```python
from build123d import *

# Parameters (mm, degrees)
SKETCH1_W           = 60
SKETCH1_H           = 60
SKETCH1_R           = 28
SKETCH1_R_2         = 2.5
BOSS_EXTRUDE1_DEPTH = 7.5
SKETCH2_W           = 83.422483418
SKETCH2_H           = 79.797227822
SKETCH2_R           = 30
CUT_EXTRUDE1_DEPTH  = 2.5
BOSS_EXTRUDE2_START = -2
BOSS_EXTRUDE2_DEPTH = 2
FILLET1_R           = 3
FILLET2_R           = 5


with BuildPart() as part:
    # Sketch1 → Boss-Extrude1 (new, symmetric)
    with BuildSketch(Plane.XY):
        Rectangle(SKETCH1_W, SKETCH1_H)
        Circle(SKETCH1_R, mode=Mode.SUBTRACT)
        with Locations((25, 25)):
            Circle(SKETCH1_R_2, mode=Mode.SUBTRACT)
        with Locations((-25, 25)):
            Circle(SKETCH1_R_2, mode=Mode.SUBTRACT)
        with Locations((-25, -25)):
            Circle(SKETCH1_R_2, mode=Mode.SUBTRACT)
        with Locations((25, -25)):
            Circle(SKETCH1_R_2, mode=Mode.SUBTRACT)
    extrude(amount=BOSS_EXTRUDE1_DEPTH, both=True)

    # Sketch2 → Cut-Extrude1 (cut, symmetric)
    with BuildSketch(Plane.XY):
        Rectangle(SKETCH2_W, SKETCH2_H)
        Circle(SKETCH2_R, mode=Mode.SUBTRACT)
    extrude(amount=CUT_EXTRUDE1_DEPTH, both=True, mode=Mode.SUBTRACT)

    # Sketch3 → Boss-Extrude2 (add)
    with BuildSketch(Plane.XY.offset(7.5).offset(BOSS_EXTRUDE2_START)):
        with BuildLine():
            Line((14.986146269, -0.644530834), (22.978250586, -16))
            ThreePointArc((22.978250586, -16), (23.61864626, -15.038601957), (24.218842251, -14.051607738))
            Line((24.218842251, -14.051607738), (13.465479299, 6.609150267))
            Line((13.465479299, 6.609150267), (13.13845395, 7.237473855))
            ThreePointArc((13.13845395, 7.237473855), (7.905893272, 12.747425292), (0.644530834, 14.986146269))
            Line((0.644530834, 14.986146269), (16, 22.978250586))
            ThreePointArc((16, 22.978250586), (15.038601957, 23.61864626), (14.051607738, 24.218842251))
            Line((14.051607738, 24.218842251), (-7.237473855, 13.13845395))
            ThreePointArc((-7.237473855, 13.13845395), (-12.747425292, 7.905893272), (-14.986146269, 0.644530834))
            Line((-14.986146269, 0.644530834), (-22.978250586, 16))
            ThreePointArc((-22.978250586, 16), (-23.61864626, 15.038601957), (-24.218842251, 14.051607738))
            Line((-24.218842251, 14.051607738), (-13.465479299, -6.609150267))
            Line((-13.465479299, -6.609150267), (-13.13845395, -7.237473855))
            ThreePointArc((-13.13845395, -7.237473855), (-7.905893272, -12.747425292), (-0.644530834, -14.986146269))
            Line((-0.644530834, -14.986146269), (-16, -22.978250586))
            ThreePointArc((-16, -22.978250586), (-15.038601957, -23.61864626), (-14.051607738, -24.218842251))
            Line((-14.051607738, -24.218842251), (6.609150267, -13.465479299))
            Line((6.609150267, -13.465479299), (7.237473855, -13.13845395))
            ThreePointArc((7.237473855, -13.13845395), (12.747425292, -7.905893272), (14.986146269, -0.644530834))
        make_face()
    extrude(amount=BOSS_EXTRUDE2_DEPTH)

    # Fillet1
    fillet1_edges = [part.edges().sort_by_distance(p)[0] for p in [
        (24.218842251, -14.051607738, 6.5),
        (22.978250586, -16, 6.5),
        (14.986146269, -0.644530834, 6.5),
        (-14.051607738, -24.218842251, 6.5),
        (-16, -22.978250586, 6.5),
        (-0.644530834, -14.986146269, 6.5),
        (-24.218842251, 14.051607738, 6.5),
        (-22.978250586, 16, 6.5),
        (-14.986146269, 0.644530834, 6.5),
        (14.051607738, 24.218842251, 6.5),
        (16, 22.978250586, 6.5),
        (0.644530834, 14.986146269, 6.5),
    ]]
    fillet(fillet1_edges, radius=FILLET1_R)

    # Fillet2
    fillet2_edges = [part.edges().sort_by_distance(p)[0] for p in [
        (30, -30, -5),
        (-30, -30, -5),
        (-30, 30, -5),
        (30, 30, -5),
        (30, -30, 5),
        (-30, -30, 5),
        (-30, 30, 5),
        (30, 30, 5),
    ]]
    fillet(fillet2_edges, radius=FILLET2_R)


solid = part.part
```
For this review, take the finished solid that the model builds, in its own axes (mm). A direction names the side the tool comes from. Coordinates: 2 decimals unless noted, no trailing zeros. Write each loop counter-clockwise with the first axis right and the second up, starting at its lowest first coordinate (ties: lowest second). Pieces come first, ordered by that corner, then holes. Notation, with made-up numbers: (7.25, -31.75) -> (34.25, -31.75) arc R20 ccw to (34.25, -19.75) -> close; hole circle Ø8 at (30, -23.75). An arc over 180 degrees is marked (long way). Put each result on its own line as item: value.
Q1. Clearance check with a flat-ended pin moving along its axis: pin 1 Ø9 at (x, y) = (12, -9.5) entering from -Z. State where the tip first meets the part, or that it passes through.
From the geometry:
pin 1: stops at z = 5.5
Q2. Take a section at A-A, the plane z = -5.75. State the section outline as (x, y) points.
From the geometry:
outline: (-30, -25) arc R5 ccw to (-25, -30) -> (25, -30) arc R5 ccw to (30, -25) -> (30, 25) arc R5 ccw to (25, 30) -> (-25, 30) arc R5 ccw to (-30, 25) -> close; hole circle Ø56 at (0, 0); hole circle Ø5 at (-25, -25); hole circle Ø5 at (-25, 25); hole circle Ø5 at (25, -25); hole circle Ø5 at (25, 25)
Q3. Take a section at C-C, the plane x = -26. Count the separate pieces of the cut face and the enclosed holes in it, then the cut area to 3 significant figures.
From the geometry:
separate pieces: 6
enclosed holes: 0
area: 346 mm2
Q4. Take a section at D-D, the plane y = 11. State the section outline as (x, z) points, then the cut area to 3 significant figures.
From the geometry:
outline: (-30, -7.5) -> (-25.75, -7.5) -> (-25.75, 5.5) -> (-20.38, 5.5) -> (-20.38, 7.5) -> (-30, 7.5) -> (-30, 2.5) -> (-27.91, 2.5) -> (-27.91, -2.5) -> (-30, -2.5) -> close; (-10.2, 5.5) -> (10.2, 5.5) -> (10.2, 7.5) -> (-10.2, 7.5) -> close; (25.75, -7.5) -> (30, -7.5) -> (30, -2.5) -> (27.91, -2.5) -> (27.91, 2.5) -> (30, 2.5) -> (30, 7.5) -> (25.75, 7.5) -> close
area: 158 mm2
Q5. The part is to be moulded in two halves that separate along Y. For faces 1 (the cylindrical face through (24.67, 27.48, 4.96)), 2 (the cylindrical face through (10.641, 10.572, 6.486)), 3 (the cylindrical face through (28, -29, -5)), 4 (the cylindrical face through (-29, 28, 5)), say which applies: +Y half, -Y half, draft (parallel to the pull), parting line (faces both ways), or undercut.
From the geometry:
face 1: undercut
face 2: undercut
face 3: -Y half
face 4: +Y half
Q6. Wall thickness on L1, parallel to Y at x = -25, z = 4.05; L2, parallel to Y at x = -22, z = 6.5: over which ranges is each line inside the solid? List them lowest first.
From the geometry:
L1: y = -30 to -27.5, -22.5 to -12.61, 12.61 to 22.5, 27.5 to 30
L2: y = -30 to -17.32, 9.34 to 14.12, 17.29 to 30
Q7. Take a section at B-B, the plane x = -19.5. State the section outline as (y, z) points.
From the geometry:
outline: (-30, -7.5) -> (-20.09, -7.5) -> (-20.09, 7.5) -> (-30, 7.5) -> (-30, 2.5) -> (-22.8, 2.5) -> (-22.8, -2.5) -> (-30, -2.5) -> close; (4.99, 5.5) -> (9.32, 5.5) -> (9.32, 7.5) -> (4.99, 7.5) -> close; (20.09, -7.5) -> (30, -7.5) -> (30, -2.5) -> (22.8, -2.5) -> (22.8, 2.5) -> (30, 2.5) -> (30, 7.5) -> (20.09, 7.5) -> close
Q8. Tool access review of faces 5 (the flat face through (-23, 23, 2.5)), 6 (the flat face through (-23, -23, 2.5)), 7 (the cylindrical face through (24.313, -10.066, 6.514)), 8 (the flat face through (23, -23, -2.5)): name each direction out of +Z, -Z, +X, -X, +Y, -Y from which nothing blocks a thin tool from reaching the whole face with its end or side.
From the geometry:
face 5: -X, +Y
face 6: -X, -Y
face 7: +Z, -Z
face 8: +X, -Y
